Could you check a few things on this model? Use its own coordinates, in mm. Face numbers are marked on the shaded views. A direction names the side the tool comes from. Round coordinates to 2 decimals unless told otherwise and drop trailing zeros. Loops run counter-clockwise (first coordinate to the right, second up) from the corner with the lowest first, then second, coordinate; pieces in that order, holes last. Notation, with made-up numbers: (36, 17.5) -> (43, 17.5) arc R29 cw to (43, 49.5) -> close; hole circle Ø9 at (17.5, -7.5). An arc over 180 degrees is marked (long way). One line per item, written item: value.
Autodesk Inventor part; units mm, degrees
ref_plane "YZ Plane" through (0, 0, 0) normal (1, 0, 0) x (0, 1, 0)
ref_plane "XZ Plane" through (0, 0, 0) normal (0, 1, 0) x (-1, 0, 0)
ref_plane "XY Plane" through (0, 0, 0) normal (0, 0, 1) x (1, 0, 0)
sketch "Sketch1" plane through (0, 0, 0) normal (0, 0, 1) x (1, 0, 0)
  circle A0 centre (0, 0) radius 20
  dimension "d0" = 40
extrude "Extrusion1" add sketch "Sketch1" along normal blind 24
sketch "Sketch2" plane through (0, 0, 24) normal (0, 0, 1) x (1, 0, 0)
  arc A0 (-9.5263, 5.5) -> (-9.5263, -5.5) centre (0, 0) ccw
  line L0 (-9.5263, 5.5) -> (-17.3205, 10)
  circle A1 centre (0, 0) radius 20
  line L1 (0, 0) -> (20, 0) construction
  line L2 (-9.5263, -5.5) -> (-17.3205, -10)
  line L3 (0, 0) -> (20, 0) construction
  line L4 (0, 0) -> (0, 20) construction
  arc A2 (9.5263, -5.5) -> (9.5263, 5.5) centre (0, 0) ccw
  line L5 (9.5263, 5.5) -> (17.3205, 10)
  line L6 (9.5263, -5.5) -> (17.3205, -10)
  dimension "d3" = 22
  dimension "d4" = 150
  dimension "d5" = 150
extrude "Extrusion2" add sketch "Sketch2" along normal blind 17 contours A0 L2 A1 L0 | A1 L6 A2 L5
sketch "Sketch3" plane through (0, 0, 24) normal (0, 0, 1) x (1, 0, 0)
  circle A0 centre (0, 0) radius 10
  dimension "d8" = 20
extrude "Extrusion3" cut sketch "Sketch3" against normal through all
properties part number "22MM JAW"
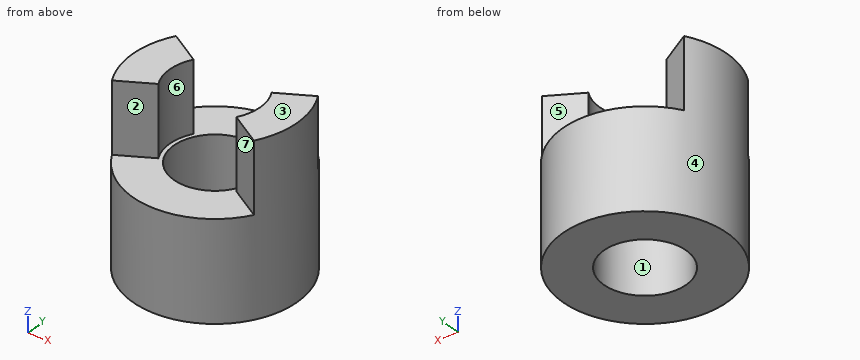
(1) If I drill on L1, parallel to Y at x = 0, z = 12; L2, parallel to Z at x = 9, y = -12.5; L3, parallel to X at y = 8, z = 19, over which ranges is the centre line in solid material (lowest first)?
Recorded:
L1: -20 to -10, 10 to 20
L2: 0 to 24
L3: -18.33 to -6, 6 to 18.33
(2) If we section it at A-A, the plane x = 0: Please give me the cut outline in (y, z).
Recorded:
outline: (-20, 0) -> (-10, 0) -> (-10, 24) -> (-20, 24) -> close; (10, 0) -> (20, 0) -> (20, 24) -> (10, 24) -> close
(3) If we section it at C-C, the plane y = -8: Please give me the cut outline in (x, z), then the cut area to 3 significant figures.
Recorded:
outline: (-18.33, 0) -> (-6, 0) -> (-6, 24) -> (-13.86, 24) -> (-13.86, 41) -> (-18.33, 41) -> close; (6, 0) -> (18.33, 0) -> (18.33, 41) -> (13.86, 41) -> (13.86, 24) -> (6, 24) -> close
area: 744 mm²
(4) Thinking about a two-plate mould opening in Y: for the marked faces 1, 2 and 3, which applies, released by +Y, released by -Y, zero draft, split by the parting line, or undercut?
Recorded:
face 1: undercut
face 2: released by -Y
face 3: zero draft
(5) If we section it at B-B, the plane z = 37: Please give me the cut outline in (x, y), then the cut area to 3 significant figures.
Recorded:
outline: (-17.32, -10) -> (-9.53, -5.5) arc R11 cw to (-9.53, 5.5) -> (-17.32, 10) arc R20 ccw to start; (9.53, -5.5) -> (17.32, -10) arc R20 ccw to (17.32, 10) -> (9.53, 5.5) arc R11 cw to start
area: 292 mm²
(6) I'm going to push flat-ended pins straight in: pin 1 Ø8 at (x, z) = (-10.5, 10) entering from -Y; pin 2 Ø5 at (x, z) = (8, 15) entering from +Y; pin 3 Ø2 at (x, z) = (-9.5, 25.5) entering from +Y. Where does each tip first touch, or does it pass through?
Recorded:
pin 1: y = -18.91
pin 2: y = 19.23
pin 3: y = 6.06
(7) If we section it at D-D, the plane x = -15: Please give me the cut outline in (y, z), then the cut area to 3 significant figures.
Recorded:
outline: (-13.23, 0) -> (13.23, 0) -> (13.23, 24) -> (8.66, 24) -> (8.66, 41) -> (-8.66, 41) -> (-8.66, 24) -> (-13.23, 24) -> close
area: 929 mm²
(8) For the marked faces 4, 5, 6 and 7, which set-ups out of +Z, -Z, +X, -X, +Y, -Y let a thin tool reach every point of the face, with its end or its side?
Recorded:
face 4: +Z, -Z
face 5: +Z, +Y
face 6: +Z
face 7: +Z, -Y
